```python
from build123d import *

# Parameters (mm, degrees)
SKETCH2_W           = 42
SKETCH2_H           = 42
SKETCH2_R           = 2
BOSS_EXTRUDE3_DEPTH = 5.5
SKETCH5_W           = 42
SKETCH5_H           = 42
SKETCH5_R           = 2
SKETCH5_R_2         = 5
BOSS_EXTRUDE5_DEPTH = 2


with BuildPart() as part:
    # Sketch2 → Boss-Extrude3 (new body)
    with BuildSketch(Plane.XY):
        with Locations((17.05217694, 12.5)):
            Rectangle(SKETCH2_W, SKETCH2_H)
        with Locations((1.05217694, 28.5)):
            Circle(SKETCH2_R, mode=Mode.SUBTRACT)
        with Locations((1.05217694, -3.5)):
            Circle(SKETCH2_R, mode=Mode.SUBTRACT)
        with Locations((33.05217694, -3.5)):
            Circle(SKETCH2_R, mode=Mode.SUBTRACT)
        with Locations((33.05217694, 28.5)):
            Circle(SKETCH2_R, mode=Mode.SUBTRACT)
    extrude(amount=BOSS_EXTRUDE3_DEPTH)

    # Sketch5 → Boss-Extrude5 (add)
    with BuildSketch(Plane.XY.offset(5.5)):
        with Locations((17.05217694, 12.5)):
            Rectangle(SKETCH5_W, SKETCH5_H)
        with Locations((1.05217694, 28.5)):
            Circle(SKETCH5_R, mode=Mode.SUBTRACT)
        with Locations((33.05217694, 28.5)):
            Circle(SKETCH5_R, mode=Mode.SUBTRACT)
        with Locations((1.05217694, -3.5)):
            Circle(SKETCH5_R, mode=Mode.SUBTRACT)
        with Locations((33.05217694, -3.5)):
            Circle(SKETCH5_R, mode=Mode.SUBTRACT)
        with Locations((17.05217694, 11.592136271)):
            Circle(SKETCH5_R_2, mode=Mode.SUBTRACT)
    extrude(amount=BOSS_EXTRUDE5_DEPTH)


solid = part.part
```
Can you work these out from the model? Positions are in its coordinate system, mm. A direction names the side the tool comes from. Round coordinates to 2 decimals unless told otherwise and drop trailing zeros. Order: outer loops, then holes, each group sorted by start corner. A loop starts at its lowest first (then second) coordinate and runs counter-clockwise, first axis right, second up. Notation, with made-up numbers: (15.25, 50.5) -> (48.25, 50.5) arc R21 cw to (48.25, 83.5) -> close; hole circle Ø11 at (32.25, 83). An arc over 180 degrees is marked (long way). Return JSON: item names as keys, results as strings. Group by question number.
1. If we section it at B-B, the plane z = 3.75: Write out the boundary of the cut face in (x, y).
2. If we section it at C-C, the plane x = 21.5: Write out the boundary of the cut face in (y, z), then the cut area to 3 significant figures.
3. Will these pins go through, and if not, where does the flat tip stop? pin 1 (8 mm diameter, centred on x = 20, y = 16.5, fed in from -Z); pin 2 (9 mm diameter, centred on x = 17.05, y = 11.59, fed in from +Z).
4. Which directions (+Z, -Z, +X, -X, +Y, -Y) give clear straight access to the entire face, cutting with the end or side of a thin tool? Please do faces 4 (the face through (17, 12, 5.5)), 5 (the face through (0.619, 26.548, 3.698)).
5. We'd pull the mould along X, two halves only. Please class faces 1 (the face through (-3.948, 12, 4)), 2 (the face through (17, -8.5, 4)), 3 (the face through (34.9, -4.27, 3.7)): released by +X, released by -X, zero draft, split by the parting line, or undercut.
6. If we section it at A-A, the plane y = -3.5: Write out the boundary of the cut face in (x, z).
7. I need wall thicknesses on line 1 (Y direction, x = -0.5, z = 4.5); line 2 (Y direction, x = 0, z = 0.75); line 3 (Z direction, x = 20, y = 9). Which ranges of each line are inside material? Lowest first, please. Write a range as [from, to].
Output values:
{
 "1": {"outline": "(-3.95, -8.5) -> (38.05, -8.5) -> (38.05, 33.5) -> (-3.95, 33.5) -> close; hole circle Ø4 at (1.05, -3.5); hole circle Ø4 at (1.05, 28.5); hole circle Ø4 at (33.05, -3.5); hole circle Ø4 at (33.05, 28.5)"},
 "2": {"outline": "(-8.5, 0) -> (33.5, 0) -> (33.5, 7.5) -> (13.88, 7.5) -> (13.88, 5.5) -> (9.31, 5.5) -> (9.31, 7.5) -> (-8.5, 7.5) -> close", "area": "306 mm²"},
 "3": {"pin 1": "z = 0", "pin 2": "z = 5.5"},
 "4": {"face 4": "+Z", "face 5": "+Z, -Z"},
 "5": {"face 1": "released by -X", "face 2": "zero draft", "face 3": "undercut"},
 "6": {"outline": "(-3.95, 0) -> (-0.95, 0) -> (-0.95, 7.5) -> (-3.95, 7.5) -> close; (3.05, 0) -> (31.05, 0) -> (31.05, 7.5) -> (3.05, 7.5) -> close; (35.05, 0) -> (38.05, 0) -> (38.05, 7.5) -> (35.05, 7.5) -> close"},
 "7": {"line 1": "[-8.5, -4.76], [-2.24, 27.24], [29.76, 33.5]", "line 2": "[-8.5, -5.2], [-1.8, 26.8], [30.2, 33.5]", "line 3": "[0, 5.5]"}
}
